Geometry check sheet. Reference: drawing and pictorial views, mm from the part's lowest x, y, z. A direction names the side the tool comes from. Coordinates: 2 decimals unless noted, no trailing zeros. Write each loop counter-clockwise with the first axis right and the second up, starting at its lowest first coordinate (ties: lowest second). Pieces come first, ordered by that corner, then holes. Notation, with made-up numbers: (-19, -17) - (19, -17) arc R19 ccw to (19, -7) - close; hole circle Ø2 at (33, 33.25). An arc over 180 degrees is marked (long way). Use one line per item in the form item = value. Start each with the question number.
(1) Sectioned sample at D-D (z = 1.5). Record the cut outline in (x, y).
(2) Tool access check on the marked faces 1, 2, 3, 4 and 5. Record the directions out of +Z, -Z, +X, -X, +Y, -Y that give a thin tool (end or side, any length) a straight path to the whole face; none if there is none.
(3) Material ranges on line 1 (X direction, y = 17, z = 8); line 2 (Y direction, x = 63, z = 1.75); line 3 (Y direction, x = 52.5, z = 11.25), recorded low to high. Write a range as [from, to].
(4) Sectioned sample at A-A (y = 34.5). Record the cut outline in (x, z), and give its area (3 significant figures).
(5) Gauge pin test, flat ends, axial feed: pin 1 Ø2.5 at (y, z) = (33, 9.5) entering from -X; pin 2 Ø7 at (x, z) = (70, 4) entering from +Y; pin 3 Ø4 at (x, z) = (2.5, 10.5) entering from +Y. Record the tip position at first contact, or that the pin passes through.
(6) Sectioned sample at C-C (x = 47.57). Record the cut outline in (y, z).
(7) Mould release check, pull along X, two halves, no side actions. Record for the marked faces 6, 7, 8 and 9: released by +X, released by -X, zero draft, split by the parting line, or undercut.
(8) Sectioned sample at B-B (z = 8). Record the cut outline in (x, y).
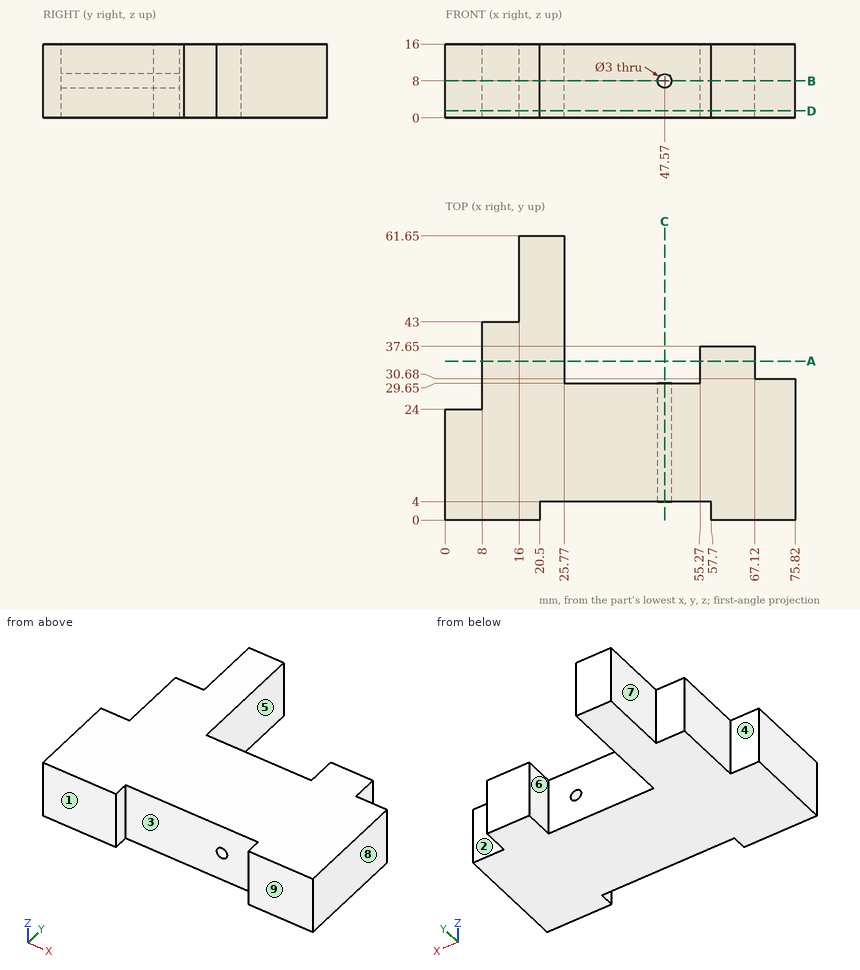
Answers below:
q1.outline = (0, 0) - (20.5, 0) - (20.5, 4) - (57.7, 4) - (57.7, 0) - (75.82, 0) - (75.82, 30.68) - (67.12, 30.68) - (67.12, 37.65) - (55.27, 37.65) - (55.27, 29.65) - (25.77, 29.65) - (25.77, 61.65) - (16, 61.65) - (16, 43) - (8, 43) - (8, 24) - (0, 24) - close
q2.face_1 = +Z, -Z, +X, -X, -Y
q2.face_2 = +Z, -Z, +X, +Y
q2.face_3 = +Z, -Z, -Y
q2.face_4 = +Z, -Z, -X, +Y
q2.face_5 = +Z, -Z, +Y
q3.line_1 = [0, 46.07], [49.07, 75.82]
q3.line_2 = [0, 37.65]
q3.line_3 = [4, 29.65]
q4.outline = (8, 0) - (25.77, 0) - (25.77, 16) - (8, 16) - close; (55.27, 0) - (67.12, 0) - (67.12, 16) - (55.27, 16) - close
q4.area = 474 mm2
q5.pin_1 = 8
q5.pin_2 = 37.65
q5.pin_3 = 24
q6.outline = (4, 0) - (29.65, 0) - (29.65, 6.5) - (4, 6.5) - close; (4, 9.5) - (29.65, 9.5) - (29.65, 16) - (4, 16) - close
q7.face_6 = undercut
q7.face_7 = released by -X
q7.face_8 = released by +X
q7.face_9 = zero draft
q8.outline = (0, 0) - (20.5, 0) - (20.5, 4) - (46.07, 4) - (46.07, 29.65) - (25.77, 29.65) - (25.77, 61.65) - (16, 61.65) - (16, 43) - (8, 43) - (8, 24) - (0, 24) - close; (49.07, 4) - (57.7, 4) - (57.7, 0) - (75.82, 0) - (75.82, 30.68) - (67.12, 30.68) - (67.12, 37.65) - (55.27, 37.65) - (55.27, 29.65) - (49.07, 29.65) - close
